For this review, use the dimensioned drawing (mm, ordinates from the lowest corner) and the shaded views. A direction names the side the tool comes from. Coordinates: 2 decimals unless noted, no trailing zeros. Write each loop counter-clockwise with the first axis right and the second up, starting at its lowest first coordinate (ties: lowest second). Pieces come first, ordered by that corner, then holes. Notation, with made-up numbers: M 3.5,18 L 18.5,18 A27 cw 18.5,55 Z; hole C 33.25,-25.75 d7. An arc over 180 degrees is marked long. One line per question, with ' | ' between items.
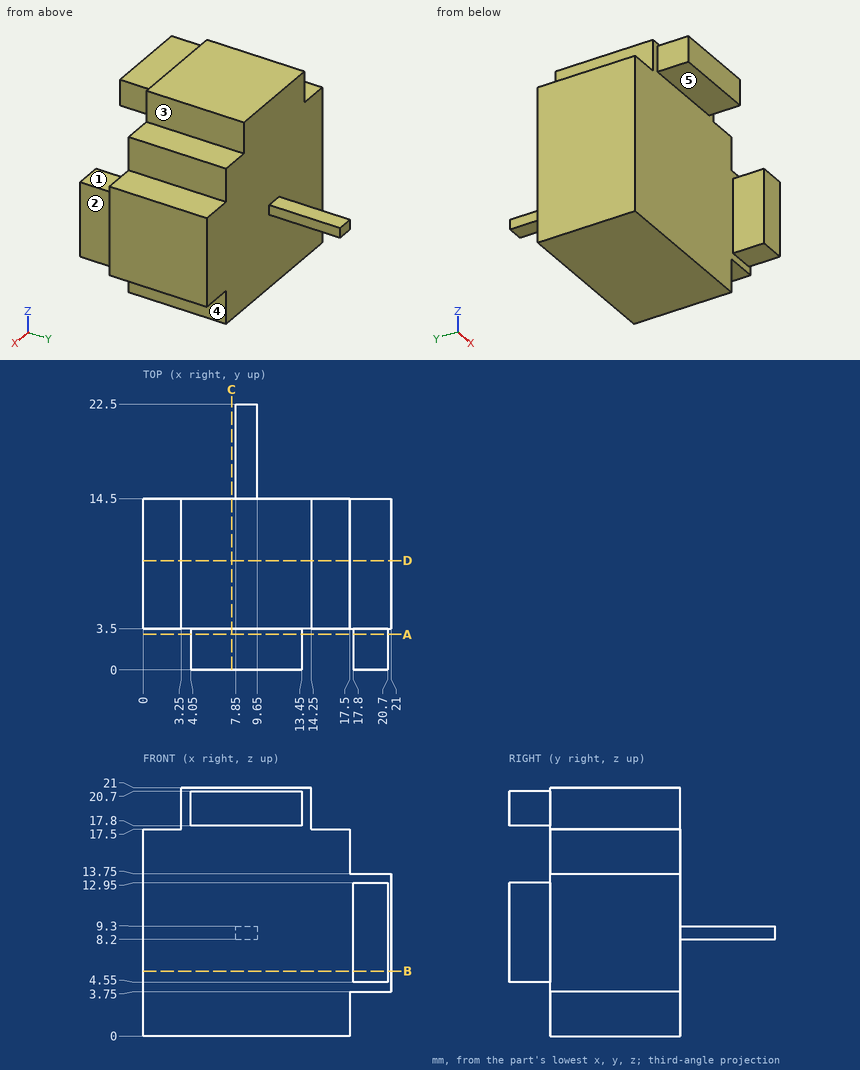
1. Insertion check: pin 1 Ø3 at (x, y) = (17, 15.5) entering from -Z; pin 2 Ø1.8 at (y, z) = (2, 9) entering from +X; pin 3 Ø1 at (y, z) = (6.5, 20) entering from -X; pin 4 Ø6.5 at (x, z) = (12, 15) entering from +Y. Each pin has a flat end and moves straight along its axis. Give the tip position at first contact, or say it passes through.
Answer sheet:
pin 1: z = 0 | pin 2: x = 20.7 | pin 3: x = 3.25 | pin 4: y = 14.5
2. Take a section at C-C (x = 7.5). Write out the cut boundary in (y, z), then the cut area to 3 significant figures.
Answer sheet:
outline: M 0,17.8 L 3.5,17.8 L 3.5,0 L 14.5,0 L 14.5,21 L 3.5,21 L 3.5,20.7 L 0,20.7 Z | area: 241 mm^2
3. Tool access review of the marked faces 1, 2, 3, 4 and 5: name each direction out of +Z, -Z, +X, -X, +Y, -Y from which nothing blocks a thin tool from reaching the whole face with its end or side.
Answer sheet:
face 1: +Z, +X, -X, -Y | face 2: +Z, -Z, +X, -Y | face 3: +Z, +X, +Y, -Y | face 4: -Z, +X, +Y, -Y | face 5: -Z, +X, -X, -Y
4. Take a section at A-A (y = 3). Write out the cut boundary in (x, z), then the cut area to 3 significant figures.
Answer sheet:
outline: M 4.05,17.8 L 13.45,17.8 L 13.45,20.7 L 4.05,20.7 Z; M 17.8,4.55 L 20.7,4.55 L 20.7,12.95 L 17.8,12.95 Z | area: 51.6 mm^2
5. Take a section at D-D (y = 9.25). Write out the cut boundary in (x, z), then the cut area to 3 significant figures.
Answer sheet:
outline: M 0,0 L 17.5,0 L 17.5,3.75 L 21,3.75 L 21,13.75 L 17.5,13.75 L 17.5,17.5 L 14.25,17.5 L 14.25,21 L 3.25,21 L 3.25,17.5 L 0,17.5 Z | area: 380 mm^2
6. To check wall thickness, follow line 1 along X through (y, z) = (4, 2.5); line 2 along Z through (x, y) = (19, 5.5). State the ranges of each line that lie inside material, in increasing order. Write a range as [from, to].
Answer sheet:
line 1: [0, 17.5] | line 2: [3.75, 13.75]
7. Take a section at B-B (z = 5.5). Write out the cut boundary in (x, y).
Answer sheet:
outline: M 0,3.5 L 17.8,3.5 L 17.8,0 L 20.7,0 L 20.7,3.5 L 21,3.5 L 21,14.5 L 0,14.5 Z
